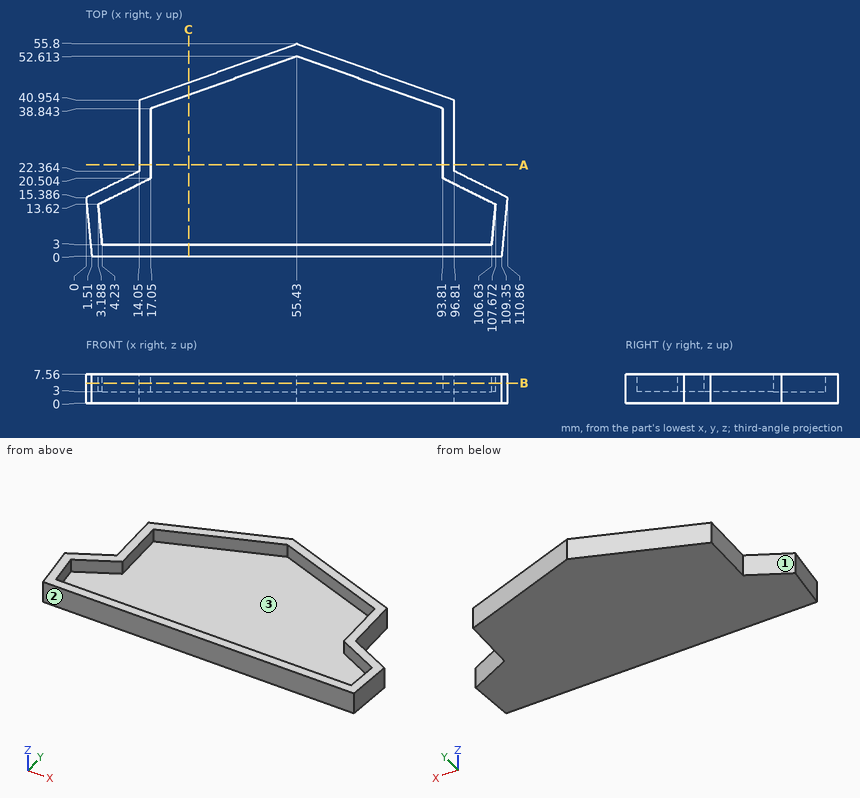
Drawing for the job (mm, zero at the part's lowest x, y, z). Round coordinates to 2 decimals unless told otherwise and drop trailing zeros. Order: outer loops, then holes, each group sorted by start corner. A loop starts at its lowest first (then second) coordinate and runs counter-clockwise, first axis right, second up.
Item 1: Saw through at C-C on x = 27. Write the cut outline in (y, z), then the cut area to 3 significant figures.
Item 2: Pin check, flat tips, straight feed: pin 1 (2 mm diameter, centred on y = 8, z = 5, fed in from +X); pin 2 (15 mm diameter, centred on x = 56, y = 20.5, fed in from +Z); pin 3 (2 mm diameter, centred on y = 13, z = 1.5, fed in from -X). Stop position of each tip, or through.
Item 3: Saw through at B-B on z = 5.25. Write the cut outline in (x, y).
Item 4: Probe line 1 along X through (y, z) = (36, 3.75); line 2 along Y through (x, z) = (39, 7) (1 decimal); line 3 along Y through (x, z) = (81, 3.75) (1 decimal). List the from-to ranges inside material, lowest first.
Item 5: Saw through at A-A on y = 24. Write the cut outline in (x, z), then the cut area to 3 significant figures.
Item 6: Mould opens along X. For the marked faces 1, 2 and 3 say: pulls with the +X half, pulls with the -X half, needs draft (parallel to the pull), parting line crosses it, or undercut.
Reported:
1. outline: (0, 0) - (45.6, 0) - (45.6, 7.56) - (42.41, 7.56) - (42.41, 3) - (3, 3) - (3, 7.56) - (0, 7.56) - close
1. area: 165 mm2
2. pin 1: stops at x = 110.23
2. pin 2: stops at z = 3
2. pin 3: stops at x = 0.14
3. outline: (0, 15.39) - (1.51, 0) - (109.35, 0) - (110.86, 15.39) - (96.81, 22.36) - (96.81, 40.95) - (55.43, 55.8) - (14.05, 40.95) - (14.05, 22.36) - close; hole (3.19, 13.62) - (4.23, 3) - (106.63, 3) - (107.67, 13.62) - (93.81, 20.5) - (93.81, 38.84) - (55.43, 52.61) - (17.05, 38.84) - (17.05, 20.5) - close
4. line 1: x = 14.05 to 17.05, 93.81 to 96.81
4. line 2: y = 0 to 3, 46.7 to 49.9
4. line 3: y = 0 to 3, 43.4 to 46.6
5. outline: (14.05, 0) - (96.81, 0) - (96.81, 7.56) - (93.81, 7.56) - (93.81, 3) - (17.05, 3) - (17.05, 7.56) - (14.05, 7.56) - close
5. area: 276 mm2
6. face 1: pulls with the -X half
6. face 2: needs draft
6. face 3: undercut
